Read the model definition and answer for the solid it produces. Units are mm, in the model's axes. A direction names the side the tool comes from. Coordinates: 2 decimals unless noted, no trailing zeros. Order: outer loops, then holes, each group sorted by start corner. A loop starts at its lowest first (then second) coordinate and runs counter-clockwise, first axis right, second up. Notation, with made-up numbers: M 33.25,-12 L 87.25,-12 A7 ccw 87.25,-6 Z; hole C 31,11.5 d4. An arc over 180 degrees is marked long. Put each result on its own line as item: value.
from build123d import *

# Parameters (mm, degrees)
SKETCH1_R           = 1.6
BOSS_EXTRUDE1_DEPTH = 8
CHAMFER1_SIZE       = 1
SKETCH2_R           = 1.6
BOSS_EXTRUDE3_DEPTH = 8
FILLET1_R           = 10
CHAMFER2_SIZE       = 1
CHAMFER3_SIZE       = 1


with BuildPart() as part:
    # Sketch1 → Boss-Extrude1 (new body)
    with BuildSketch(Plane.XY):
        with BuildLine():
            Line((-0.5, 3), (45.5, 3))
            ThreePointArc((45.5, 3), (47.267766953, 2.267766953), (48, 0.5))
            Line((48, 0.5), (48, -0.5))
            ThreePointArc((48, -0.5), (47.267766953, -2.267766953), (45.5, -3))
            Line((45.5, -3), (-0.5, -3))
            ThreePointArc((-0.5, -3), (-2.267766953, -2.267766953), (-3, -0.5))
            Line((-3, -0.5), (-3, 0.5))
            ThreePointArc((-3, 0.5), (-2.267766953, 2.267766953), (-0.5, 3))
        make_face()
        Circle(SKETCH1_R, mode=Mode.SUBTRACT)
        with Locations((7.5, 0)):
            Circle(SKETCH1_R, mode=Mode.SUBTRACT)
        with Locations((15, 0)):
            Circle(SKETCH1_R, mode=Mode.SUBTRACT)
        with Locations((22.5, 0)):
            Circle(SKETCH1_R, mode=Mode.SUBTRACT)
        with Locations((30, 0)):
            Circle(SKETCH1_R, mode=Mode.SUBTRACT)
        with Locations((37.5, 0)):
            Circle(SKETCH1_R, mode=Mode.SUBTRACT)
        with Locations((45, 0)):
            Circle(SKETCH1_R, mode=Mode.SUBTRACT)
    extrude(amount=BOSS_EXTRUDE1_DEPTH)

    # Chamfer1
    chamfer1_edges = [part.edges().sort_by_distance(p)[0] for p in [
        (-1.6, 0, 0),
        (-1.6, 0, 8),
        (5.9, 0, 0),
        (5.9, 0, 8),
        (13.4, 0, 0),
        (13.4, 0, 8),
        (20.9, 0, 0),
        (20.9, 0, 8),
        (28.4, 0, 0),
        (28.4, 0, 8),
    ]]
    chamfer(chamfer1_edges, length=CHAMFER1_SIZE)

    # Sketch2 → Boss-Extrude3 (add)
    with BuildSketch(Plane.XY.offset(8)):
        with BuildLine():
            ThreePointArc((-3, 0.5), (-2.809698831, 1.456708581), (-2.267766953, 2.267766953))
            Line((-2.267766953, 2.267766953), (-18.529200529, -13.993666623))
            ThreePointArc((-18.529200529, -13.993666623), (-19.261433576, -15.761433576), (-18.529200529, -17.529200529))
            Line((-18.529200529, -17.529200529), (-17.822093748, -18.23630731))
            ThreePointArc((-17.822093748, -18.23630731), (-16.054326795, -18.968540357), (-14.286559842, -18.23630731))
            Line((-14.286559842, -18.23630731), (0.949747468, -3))
            Line((0.949747468, -3), (-0.5, -3))
            ThreePointArc((-0.5, -3), (-2.267766953, -2.267766953), (-3, -0.5))
            Line((-3, -0.5), (-3, 0.5))
        make_face()
        with Locations((-16.054326795, -15.761433576)):
            Circle(SKETCH2_R, mode=Mode.SUBTRACT)
        with Locations((-10.751025936, -10.458132717)):
            Circle(SKETCH2_R, mode=Mode.SUBTRACT)
        with Locations((-5.447725077, -5.154831858)):
            Circle(SKETCH2_R, mode=Mode.SUBTRACT)
    extrude(amount=-BOSS_EXTRUDE3_DEPTH)

    # Fillet1
    fillet1_edges = [part.edges().sort_by_distance(p)[0] for p in [
        (0.949747468, -3, 4),
    ]]
    fillet(fillet1_edges, radius=FILLET1_R)

    # Chamfer2
    chamfer2_edges = [part.edges().sort_by_distance(p)[0] for p in [
        (-17.654326795, -15.761433576, 8),
        (-12.351025936, -10.458132717, 8),
        (-7.047725077, -5.154831858, 8),
        (-7.047725077, -5.154831858, 0),
        (-12.351025936, -10.458132717, 0),
        (-17.654326795, -15.761433576, 0),
    ]]
    chamfer(chamfer2_edges, length=CHAMFER2_SIZE)

    # Chamfer3
    chamfer3_edges = [part.edges().sort_by_distance(p)[0] for p in [
        (35.9, 0, 0),
        (35.9, 0, 8),
        (43.4, 0, 0),
        (43.4, 0, 8),
    ]]
    chamfer(chamfer3_edges, length=CHAMFER3_SIZE)


solid = part.part
Q1. A tool of negligible diameter and unlimited length cuts with its end or side. For faces 1 (the face through (26, -3, 4)), 2 (the face through (13.4, 0.07, 3.96)), from which of +Z, -Z, +X, -X, +Y, -Y can it reach the whole face along a straight path? Write none if from no direction.
Answers below:
face 1: +Z, -Z, +X, -Y
face 2: +Z, -Z
Q2. Given pin 1 (4 mm diameter, centred on x = 22.5, y = 0, fed in from +Z); pin 2 (1 mm diameter, centred on x = -11, y = -7.5, fed in from -Z); pin 3 (5 mm diameter, centred on x = -5.45, y = -5.15, fed in from +Z); pin 4 (2 mm diameter, centred on y = -6.5, z = 6, fed in from +X), each flat-ended and moving along its own axis, determine where each tip first touches the part or whether it passes through.
Answers below:
pin 1: stops at z = 7.4
pin 2: stops at z = 0
pin 3: stops at z = 7.91
pin 4: stops at x = -1.52
Q3. Find section A-A on x = 15. Write down the section's boundary in (y, z), plus the area to 3 significant figures.
Answers below:
outline: M -3,0 L -2.6,0 L -1.6,1 L -1.6,7 L -2.6,8 L -3,8 Z; M 1.6,1 L 2.6,0 L 3,0 L 3,8 L 2.6,8 L 1.6,7 Z
area: 20.4 mm^2
Q4. Consider line 1 along Y through (x, z) = (7.5, 3.8); line 2 along Y through (x, z) = (22, 5.5); line 3 along Y through (x, z) = (25, 0.75). Determine where each line is inside the solid, lowest interval first.
Answers below:
line 1: y = -3 to -1.6, 1.6 to 3
line 2: y = -3 to -1.52, 1.52 to 3
line 3: y = -3 to 3
Q5. For a pull along Y with two mould halves and no side action, classify faces 3 (the face through (47.287, -2.248, 3.944)), 4 (the face through (47.248, 2.287, 3.944)), 5 (the face through (9.2, -2.2, 0)), 6 (the face through (43.82, 1.08, 3.96)) as +Y half, -Y half, draft (parallel to the pull), parting line (faces both ways), or undercut.
Answers below:
face 3: -Y half
face 4: +Y half
face 5: draft
face 6: undercut
Q6. Find section B-B on z = 2.75. Give the number of separate pieces and of enclosed holes in the cut face, plus the area to 3 significant figures.
Answers below:
separate pieces: 1
enclosed holes: 10
area: 358 mm^2
